Verification items for the finished model (mm, model axes). Face numbers are marked on the shaded views. A direction names the side the tool comes from. Round coordinates to 2 decimals unless told otherwise and drop trailing zeros. Order: outer loops, then holes, each group sorted by start corner. A loop starts at its lowest first (then second) coordinate and runs counter-clockwise, first axis right, second up. Notation, with made-up numbers: (27.5, -7.75) -> (83.5, -7.75) arc R32 cw to (83.5, 21.25) -> close; hole circle Ø3 at (89.5, 22.25). An arc over 180 degrees is marked (long way). Put each result on its own line as item: value.
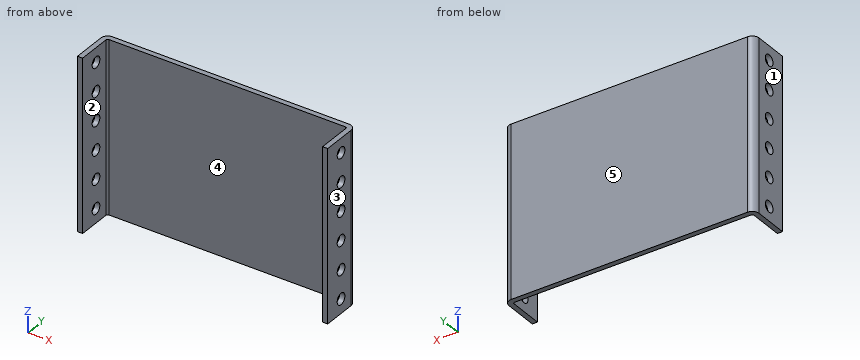
from build123d import *

# Parameters (mm, degrees)
BASE_FLANGE1_DEPTH      = 76.2
CUT_EXTRUDE1_DEPTH      = 95.858586108
CUT_EXTRUDE1_DEPTH_BACK = 95.858586108
SKETCH3_R               = 2.4892


# Sheet-metal steps are written as plain solids
with BuildPart() as part:
    # Sketch1 → Base-Flange1 (new body)
    with BuildSketch(Plane.XY):
        with BuildLine():
            Line((-53.2765, -7.9375), (-53.2765, 7.1755))
            ThreePointArc((-53.2765, 7.1755), (-53.053315367, 7.714315367), (-52.5145, 7.9375))
            Line((-52.5145, 7.9375), (52.5145, 7.9375))
            ThreePointArc((52.5145, 7.9375), (53.053315367, 7.714315367), (53.2765, 7.1755))
            Line((53.2765, 7.1755), (53.2765, -7.9375))
            Line((53.2765, -7.9375), (55.5625, -7.9375))
            Line((55.5625, -7.9375), (55.5625, 7.1755))
            ThreePointArc((55.5625, 7.1755), (54.669761469, 9.330761469), (52.5145, 10.2235))
            Line((52.5145, 10.2235), (-52.5145, 10.2235))
            ThreePointArc((-52.5145, 10.2235), (-54.669761469, 9.330761469), (-55.5625, 7.1755))
            Line((-55.5625, 7.1755), (-55.5625, -7.9375))
            Line((-55.5625, -7.9375), (-53.2765, -7.9375))
        make_face()
    extrude(amount=BASE_FLANGE1_DEPTH)

    # Sketch3 → Cut-Extrude1 (cut, two sides: drawn at the far end of the back side and taken through both)
    with BuildSketch(Plane(origin=(0, 0, 0), x_dir=(0, 0, -1), z_dir=(1, 0, 0)).offset(-CUT_EXTRUDE1_DEPTH_BACK)):
        with Locations((-6.35, 0.6985)):
            Circle(SKETCH3_R)
        with Locations((-19.05, 0.6985)):
            Circle(SKETCH3_R)
        with Locations((-31.75, 0.6985)):
            Circle(SKETCH3_R)
        with Locations((-44.45, 0.6985)):
            Circle(SKETCH3_R)
        with Locations((-57.15, 0.6985)):
            Circle(SKETCH3_R)
        with Locations((-69.85, 0.6985)):
            Circle(SKETCH3_R)
    extrude(amount=CUT_EXTRUDE1_DEPTH + CUT_EXTRUDE1_DEPTH_BACK, mode=Mode.SUBTRACT)


solid = part.part
Item 1: Section check B-B on y = 4.5. Record the boundary of the cut face in (x, z), then the cut area to 3 significant figures.
Check sheet entries:
outline: (-55.56, 0) -> (-53.28, 0) -> (-53.28, 76.2) -> (-55.56, 76.2) -> close; (53.28, 0) -> (55.56, 0) -> (55.56, 76.2) -> (53.28, 76.2) -> close
area: 348 mm^2
Item 2: Tool access check on the marked faces 4 and 5. Record the directions out of +Z, -Z, +X, -X, +Y, -Y that give a thin tool (end or side, any length) a straight path to the whole face; none if there is none.
Check sheet entries:
face 4: +Z, -Z, -Y
face 5: +Z, -Z, +X, -X, +Y
Item 3: Material ranges on L1, parallel to X at y = -1, z = 9.5; L2, parallel to Y at x = -22, z = 38; L3, parallel to Y at x = 54, z = 6, recorded low to high. Write a range as [from, to].
Check sheet entries:
L1: x = [-55.56, -53.28], [53.28, 55.56]
L2: y = [7.94, 10.22]
L3: y = [-7.94, -1.77], [3.16, 9.84]
Item 4: Gauge pin test, flat ends, axial feed: pin 1 Ø4 at (y, z) = (0.7, 44.45) entering from +X; pin 2 Ø3 at (x, z) = (-38.5, 52) entering from -Y. Record the tip position at first contact, or that the pin passes through.
Check sheet entries:
pin 1: passes through
pin 2: stops at y = 7.94
Item 5: Release check for a two-part mould opening along X. For the marked faces 1, 2 and 3 record: +X half, -X half, draft (parallel to the pull), parting line (faces both ways), or undercut.
Check sheet entries:
face 1: -X half
face 2: undercut
face 3: +X half
Item 6: Section check A-A on z = 44.45. Record the boundary of the cut face in (x, y).
Check sheet entries:
outline: (-55.56, -7.94) -> (-53.28, -7.94) -> (-53.28, -1.79) -> (-55.56, -1.79) -> close; (-55.56, 3.19) -> (-53.28, 3.19) -> (-53.28, 7.18) arc R0.76 cw to (-52.51, 7.94) -> (52.51, 7.94) arc R0.76 cw to (53.28, 7.18) -> (53.28, 3.19) -> (55.56, 3.19) -> (55.56, 7.18) arc R3.05 ccw to (52.51, 10.22) -> (-52.51, 10.22) arc R3.05 ccw to (-55.56, 7.18) -> close; (53.28, -7.94) -> (55.56, -7.94) -> (55.56, -1.79) -> (53.28, -1.79) -> close
Item 7: Section check C-C on z = 11.5. Record the boundary of the cut face in (x, y), then the cut area to 3 significant figures.
Check sheet entries:
outline: (-55.56, -7.94) -> (-53.28, -7.94) -> (-53.28, 7.18) arc R0.76 cw to (-52.51, 7.94) -> (52.51, 7.94) arc R0.76 cw to (53.28, 7.18) -> (53.28, -7.94) -> (55.56, -7.94) -> (55.56, 7.18) arc R3.05 ccw to (52.51, 10.22) -> (-52.51, 10.22) arc R3.05 ccw to (-55.56, 7.18) -> close
area: 323 mm^2
Item 8: Section check D-D on x = 25. Record the boundary of the cut face in (y, z).
Check sheet entries:
outline: (7.94, 0) -> (10.22, 0) -> (10.22, 76.2) -> (7.94, 76.2) -> close
